```python
from build123d import *

# Parameters (mm, degrees)
SKETCH1_W                        = 5.334
SKETCH1_H                        = 19.05
F_21_0_159_DIAMETER_HOLE1_D      = 4.0386
F_21_0_159_DIAMETER_HOLE1_DEPTH  = 5.334
F_21_0_159_DIAMETER_HOLE2_REACH  = 21.654
F_21_0_159_DIAMETER_HOLE2_BORE_R = 2.0193


with BuildPart() as part:
    # Sketch1 → Revolve1 (revolve)
    with BuildSketch(Plane.XY, mode=Mode.PRIVATE) as revolve1_sk:
        with Locations((2.667, 9.525)):
            Rectangle(SKETCH1_W, SKETCH1_H)
    revolve(revolve1_sk.sketch.rotate(Axis((0, 19.05, 0), (0, -1, 0)), 270), axis=Axis((0, 19.05, 0), (0, -1, 0)))

    # Sketch2 → CSK for #6 Flat Head Machine Screw (100)1 (revolve, cut)
    with BuildSketch(Plane(origin=(0, 0, 0), x_dir=(0, 0, -1), z_dir=(1, 0, 0))):
        Polygon((0, 0), (0, 19.05), (2, 19.05), (2, 10.231011227), (3.175, 9.525), (3.175, 0), align=None)
    revolve(axis=Axis((0, -6.35, 0), (0, 1, 0)), mode=Mode.SUBTRACT)

    # #21 (0.159) Diameter Hole1
    with Locations(Plane(origin=(0, 15.621, 5.334), x_dir=(1, 0, 0), z_dir=(0, 0, 1))):
        with Locations((0, 0)):
            Hole(F_21_0_159_DIAMETER_HOLE1_D / 2, depth=F_21_0_159_DIAMETER_HOLE1_DEPTH)

    # #21 (0.159) Diameter Hole2 bore (on position points) → #21 (0.159) Diameter Hole2 (cut, up to next)
    with BuildSketch(Plane(origin=(0, 3.429, 5.334), x_dir=(1, 0, 0), z_dir=(0, 0, 1)), mode=Mode.PRIVATE) as f_21_0_159_diameter_hole2_sk1:
        Circle(F_21_0_159_DIAMETER_HOLE2_BORE_R)
    f_21_0_159_diameter_hole2_tool1 = extrude(f_21_0_159_diameter_hole2_sk1.sketch, amount=-F_21_0_159_DIAMETER_HOLE2_REACH, mode=Mode.PRIVATE) & part.part
    add(f_21_0_159_diameter_hole2_tool1.solids().sort_by_distance((0, 3.429, 5.334))[0], mode=Mode.SUBTRACT)


solid = part.part
```
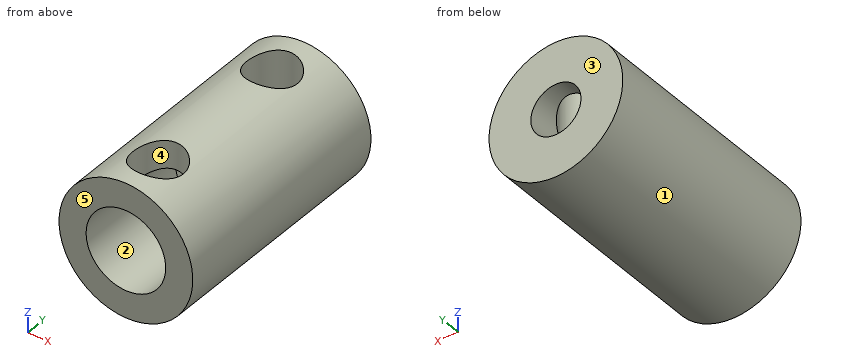
Here's how the part is built. I have some questions about the finished solid (model axes, mm). Face numbers are marked on the shaded views. A direction names the side the tool comes from. Coordinates: 2 decimals unless noted, no trailing zeros. Write each loop counter-clockwise with the first axis right and the second up, starting at its lowest first coordinate (ties: lowest second). Pieces come first, ordered by that corner, then holes. Notation, with made-up numbers: (42, 24.25) - (64, 24.25) arc R11 ccw to (64, 45.25) - close; hole circle Ø8 at (-4, 37.5). An arc over 180 degrees is marked (long way). One line per item, written item: value.
1) I'm going to push flat-ended pins straight in: P1, Ø1.5, axis at x = -2, y = 12, coming from the +Z side; P2, Ø3.5, axis at x = 0, z = 0, coming from the -Y side; P3, Ø4, axis at x = 3.5, y = 11.5, coming from the +Z side; P4, Ø3, axis at x = 0, y = 15.621, coming from the +Z side. Where does each tip first touch, or does it pass through?
Model answer:
P1: stops at z = 5.19
P2: passes through
P3: stops at z = 5.12
P4: stops at z = -1.32
2) I need wall thicknesses on line 1 along Y through (x, z) = (0, 3.6); line 2 along X through (y, z) = (14.75, 0); line 3 along X through (y, z) = (5, 0) (3 decimals). Which ranges of each line are inside material? Lowest first, please.
Model answer:
line 1: y = 0 to 1.41, 5.45 to 13.6, 17.64 to 19.05
line 2: x = -5.33 to -2, 2 to 5.33
line 3: x = -5.334 to -3.175, 3.175 to 5.334
3) Suppose I cut it at B-B on y = 12.75. Write out the boundary of the cut face in (x, z), and give its area (3 significant figures).
Model answer:
outline: circle Ø10.67 at (0, 0); hole circle Ø4 at (0, 0)
area: 76.8 mm²
4) Suppose I cut it at D-D on x = -1.25. State how many separate pieces and enclosed holes the cut face has, and give its area (3 significant figures).
Model answer:
separate pieces: 4
enclosed holes: 0
area: 92.6 mm²
5) We'd pull the mould along X, two halves only. Please class the marked faces 1, 2 and 3: pulls with the +X half, pulls with the -X half, needs draft (parallel to the pull), parting line crosses it, or undercut.
Model answer:
face 1: parting line crosses it
face 2: undercut
face 3: needs draft
6) Suppose I cut it at A-A on x = 0. Write out the boundary of the cut face in (y, z) (3 decimals), and give its area (3 significant figures).
Model answer:
outline: (0, -5.334) - (19.05, -5.334) - (19.05, -2) - (10.231, -2) - (9.525, -3.175) - (0, -3.175) - close; (0, 3.175) - (1.41, 3.175) - (1.41, 5.334) - (0, 5.334) - close; (5.448, 3.175) - (9.525, 3.175) - (10.231, 2) - (13.602, 2) - (13.602, 5.334) - (5.448, 5.334) - close; (17.64, 2) - (19.05, 2) - (19.05, 5.334) - (17.64, 5.334) - close
area: 81.6 mm²
7) Suppose I cut it at C-C on z = -3.5. Write out the boundary of the cut face in (x, y).
Model answer:
outline: (-4.03, 0) - (4.03, 0) - (4.03, 19.05) - (-4.03, 19.05) - close
8) On a 3-axis mill with a long thin cutter (end or side, diameter ignored), from which of +Z, -Z, +X, -X, +Y, -Y can I reach the whole of each face in a straight line? I mean the marked faces 4 and 5. Say none if no direction works.
Model answer:
face 4: +Z
face 5: +Z, -Z, +X, -X, -Y
